Model file for the job. Use its own axes, mm. A direction names the side the tool comes from. Round coordinates to 2 decimals unless told otherwise and drop trailing zeros. Order: outer loops, then holes, each group sorted by start corner. A loop starts at its lowest first (then second) coordinate and runs counter-clockwise, first axis right, second up. Notation, with made-up numbers: (31.25, -1.75) -> (85.25, -1.75) arc R8 ccw to (85.25, 9.25) -> close; hole circle Ø3 at (55.5, 73). An arc over 180 degrees is marked (long way). Answer as CSV lines item,"result".
```python
from build123d import *

# Parameters (mm, degrees)
SKETCH1_W           = 41.35
SKETCH1_H           = 40
BOSS_EXTRUDE1_DEPTH = 3.175
SKETCH2_W           = 3.175
SKETCH2_H           = 20.2
SKETCH2_W_2         = 15
SKETCH2_H_2         = 3.175
CUT_EXTRUDE1_DEPTH  = 4.175
SKETCH3_W           = 25
SKETCH3_H           = 26.825
CUT_EXTRUDE2_DEPTH  = 4.175


with BuildPart() as part:
    # Sketch1 → Boss-Extrude1 (new body)
    with BuildSketch(Plane(origin=(0, 0, 0), x_dir=(1, 0, 0), z_dir=(0, 1, 0))):
        with Locations((20.675, 20)):
            Rectangle(SKETCH1_W, SKETCH1_H)
    extrude(amount=BOSS_EXTRUDE1_DEPTH)

    # Sketch2 → Cut-Extrude1 (cut, through all)
    with BuildSketch(Plane.XZ):
        with Locations((39.7625, -20.1)):
            Rectangle(SKETCH2_W, SKETCH2_H)
        with Locations((1.5875, -20.1)):
            Rectangle(SKETCH2_W, SKETCH2_H)
        with Locations((20.675, -38.4125)):
            Rectangle(SKETCH2_W_2, SKETCH2_H_2)
    extrude(amount=-CUT_EXTRUDE1_DEPTH, mode=Mode.SUBTRACT)

    # Sketch3 → Cut-Extrude2 (cut, through all)
    with BuildSketch(Plane(origin=(0, 3.175, 0), x_dir=(1, 0, 0), z_dir=(0, 1, 0))):
        with Locations((20.675, 18.4125)):
            Rectangle(SKETCH3_W, SKETCH3_H)
    extrude(amount=-CUT_EXTRUDE2_DEPTH, mode=Mode.SUBTRACT)


solid = part.part
```
Q1. Saw through at C-C (y = 2.15). Write the cut outline in (x, z) (3 decimals).
Checks:
outline,"(0, -40) -> (13.175, -40) -> (13.175, -36.825) -> (28.175, -36.825) -> (28.175, -40) -> (41.35, -40) -> (41.35, -30.2) -> (38.175, -30.2) -> (38.175, -10) -> (41.35, -10) -> (41.35, 0) -> (0, 0) -> (0, -10) -> (3.175, -10) -> (3.175, -30.2) -> (0, -30.2) -> close; hole (8.175, -31.825) -> (33.175, -31.825) -> (33.175, -5) -> (8.175, -5) -> close"
Q2. Tool access for faces 4 (the flat face through (40, 2, -30.2)), 5 (the flat face through (2, 2, -30.2)), 6 (the flat face through (20, 2, -5)), 7 (the flat face through (28.175, 2, -38)): list every direction of +Z, -Z, +X, -X, +Y, -Y with a clear straight run to the whole face (end or side of a thin tool).
Checks:
face 4,"+X, +Y, -Y"
face 5,"-X, +Y, -Y"
face 6,"+Y, -Y"
face 7,"-Z, +Y, -Y"
Q3. Flat gauge pins, fed straight in: pin 1 (1 mm diameter, centred on y = 1, z = -16.5, fed in from -X) (3 decimals); pin 2 (1.5 mm diameter, centred on x = 26, z = -29.5, fed in from -Y). Where does each tip first touch, or does it go through?
Checks:
pin 1,"x = 3.175"
pin 2,"through"
Q4. Saw through at B-B (x = 31.5). Write the cut outline in (y, z) (3 decimals).
Checks:
outline,"(0, -40) -> (3.175, -40) -> (3.175, -31.825) -> (0, -31.825) -> close; (0, -5) -> (3.175, -5) -> (3.175, 0) -> (0, 0) -> close"
Q5. Wall check: L1, parallel to X at y = 1.75, z = -18 (3 decimals); L2, parallel to Z at x = 19.5, y = 0.8 (3 decimals); L3, parallel to X at y = 0.95, z = -9.5 (3 decimals). Give the ranges that are in metal, low to high. Write a range as [from, to].
Checks:
L1,"[3.175, 8.175], [33.175, 38.175]"
L2,"[-36.825, -31.825], [-5, 0]"
L3,"[0, 8.175], [33.175, 41.35]"
Q6. Saw through at A-A (z = -10.5). Write the cut outline in (x, y) (3 decimals), plus the area to 4 significant figures.
Checks:
outline,"(3.175, 0) -> (8.175, 0) -> (8.175, 3.175) -> (3.175, 3.175) -> close; (33.175, 0) -> (38.175, 0) -> (38.175, 3.175) -> (33.175, 3.175) -> close"
area,"31.75 mm²"
Q7. Mould opens along X. For faces 1 (the flat face through (3.175, 2, -20)), 2 (the flat face through (2, 2, -10)), 3 (the flat face through (20, 2, -31.825)) say: +X half, -X half, draft (parallel to the pull), parting line (faces both ways), or undercut.
Checks:
face 1,"-X half"
face 2,"draft"
face 3,"undercut"
